```python
from build123d import *

# Parameters (mm, degrees)
SKETCH_1_W           = 42.7
SKETCH_1_H           = 21
SKETCH_1_R           = 1.5
EXTRUDE_1_DEPTH      = 2
SKETCH_2_R           = 1.25
SKETCH_2_R_2         = 3
EXTRUDE_2_DEPTH      = 2
EXTRUDE_3_DEPTH      = 1
EXTRUDE_3_DEPTH_BACK = 3
SKETCH_3_W           = 42.7
SKETCH_3_H           = 21
SKETCH_4_R           = 10.5
SKETCH_4_R_2         = 1.5
EXTRUDE_4_DEPTH      = 1
FILLET_1_R           = 3
FILLET_2_R           = 5
CUT_EXTRUDE_START    = -4
SKETCH_6_R           = 1.5
CUT_EXTRUDE_1_DEPTH  = 4


with BuildPart() as part:
    # 草图1 → 凸台-拉伸1 (new body)
    with BuildSketch(Plane(origin=(0, 0, 0), x_dir=(1, 0, 0), z_dir=(0, 1, 0))):
        Rectangle(SKETCH_1_W, SKETCH_1_H)
        with Locations(Location((7.5, 5, 0), (0, 0, 270))):
            Circle(SKETCH_1_R, mode=Mode.SUBTRACT)
        with Locations(Location((7.5, -5, 0), (0, 0, 90))):
            Circle(SKETCH_1_R, mode=Mode.SUBTRACT)
        with Locations(Location((-7.5, -5, 0), (0, 0, 270))):
            Circle(SKETCH_1_R, mode=Mode.SUBTRACT)
        with Locations(Location((-7.5, 5, 0), (0, 0, 90))):
            Circle(SKETCH_1_R, mode=Mode.SUBTRACT)
        with BuildLine():
            Line((8.017950723, 1.550908082), (12.912587519, 1.550908082))
            ThreePointArc((12.912587519, 1.550908082), (14.126270768, 1.145131224), (14.697546856, 0))
            ThreePointArc((14.697546856, 0), (14.126270768, -1.145131224), (12.912587519, -1.550908082))
            Line((12.912587519, -1.550908082), (8.017950723, -1.550908082))
            add(Edge.make_bspline(
                [(0, -7.407271614), (2.092471107, -7.358009404), (3.043739342, -2.951912586), (6.007732496, -1.626733157), (8.017950723, -1.550908082)],
                knots=[0, 0, 0, 0, 0.496822763, 1, 1, 1, 1], degree=3))
            add(Edge.make_bspline(
                [(0, -7.407271614), (-2.092471107, -7.358009404), (-3.043739342, -2.951912586), (-6.007732496, -1.626733157), (-8.017950723, -1.550908082)],
                knots=[0, 0, 0, 0, 0.496822763, 1, 1, 1, 1], degree=3))
            Line((-8.017950723, -1.550908082), (-12.912587519, -1.550908082))
            ThreePointArc((-12.912587519, -1.550908082), (-14.126270768, -1.145131224), (-14.697546856, 0))
            ThreePointArc((-14.697546856, 0), (-14.126270768, 1.145131224), (-12.912587519, 1.550908082))
            Line((-12.912587519, 1.550908082), (-8.017950723, 1.550908082))
            add(Edge.make_bspline(
                [(0, 7.407271614), (-2.092471107, 7.358009404), (-3.043739342, 2.951912586), (-6.007732496, 1.626733157), (-8.017950723, 1.550908082)],
                knots=[0, 0, 0, 0, 0.496822763, 1, 1, 1, 1], degree=3))
            add(Edge.make_bspline(
                [(0, 7.407271614), (2.092471107, 7.358009404), (3.043739342, 2.951912586), (6.007732496, 1.626733157), (8.017950723, 1.550908082)],
                knots=[0, 0, 0, 0, 0.496822763, 1, 1, 1, 1], degree=3))
        make_face(mode=Mode.SUBTRACT)
    extrude(amount=EXTRUDE_1_DEPTH)

    # 草图2 → 凸台-拉伸2 (add)
    with BuildSketch(Plane.ZY.offset(21.35)):
        with BuildLine():
            Line((-10.5, 2), (-10.5, 32))
            ThreePointArc((-10.5, 32), (0, 42.5), (10.5, 32))
            Line((10.5, 32), (10.5, 2))
            Line((10.5, 2), (-10.5, 2))
        make_face()
        with Locations((0, 24.65)):
            Circle(SKETCH_2_R, mode=Mode.SUBTRACT)
        with Locations((-7.35, 32)):
            Circle(SKETCH_2_R, mode=Mode.SUBTRACT)
        with Locations((0, 39.35)):
            Circle(SKETCH_2_R, mode=Mode.SUBTRACT)
        with Locations((7.35, 32)):
            Circle(SKETCH_2_R, mode=Mode.SUBTRACT)
        with Locations((0, 32)):
            Circle(SKETCH_2_R_2, mode=Mode.SUBTRACT)
    extrude_2 = extrude(amount=-EXTRUDE_2_DEPTH)

    # 镜向1: 凸台-拉伸2 across plane
    add(extrude_2.mirror(Plane(origin=(0, 0, 0), x_dir=(0, 0, 1), z_dir=(1, 0, 0))))

    # 草图3 → 凸台-拉伸3 (add, two sides: drawn at the far end of the back side and taken through both)
    with BuildSketch(Plane.XZ.offset(-EXTRUDE_3_DEPTH_BACK)):
        Rectangle(SKETCH_3_W, SKETCH_3_H)
    extrude(amount=EXTRUDE_3_DEPTH + EXTRUDE_3_DEPTH_BACK)

    # 草图4 → 凸台-拉伸4 (add)
    with BuildSketch(Plane.XZ.offset(1)):
        with Locations(Location((0, 0, 0), (0, 0, 270))):
            Circle(SKETCH_4_R)
        with Locations(Location((0, 7, 0), (0, 0, 270))):
            Circle(SKETCH_4_R_2, mode=Mode.SUBTRACT)
        with Locations(Location((0, -7, 0), (0, 0, 270))):
            Circle(SKETCH_4_R_2, mode=Mode.SUBTRACT)
    extrude(amount=EXTRUDE_4_DEPTH)

    # 圆角1
    fillet_1_edges = [part.edges().sort_by_distance(p)[0] for p in [
        (19.35, 3, 0),
        (-19.35, 3, 0),
    ]]
    fillet(fillet_1_edges, radius=FILLET_1_R)

    # 圆角2
    fillet_2_edges = [part.edges().sort_by_distance(p)[0] for p in [
        (-21.35, -1, 0),
        (21.35, -1, 0),
    ]]
    fillet(fillet_2_edges, radius=FILLET_2_R)

    # 草图6 → 切除-拉伸1 (cut)
    with BuildSketch(Plane.XZ.offset(1).offset(CUT_EXTRUDE_START)):
        with Locations(Location((0, 7, 0), (0, 0, 270))):
            Circle(SKETCH_6_R)
        with Locations(Location((0, -7, 0), (0, 0, 270))):
            Circle(SKETCH_6_R)
    extrude(amount=CUT_EXTRUDE_1_DEPTH, mode=Mode.SUBTRACT)


solid = part.part
```
Geometry check sheet. Reference: the model listing, model coordinates, mm. A direction names the side the tool comes from. Coordinates: 2 decimals unless noted, no trailing zeros. Order: outer loops, then holes, each group sorted by start corner. A loop starts at its lowest first (then second) coordinate and runs counter-clockwise, first axis right, second up.
Item 1: Section check A-A (y = 24.65). Enter the section's corners in (x, z), plus the area to 3 significant figures.
Item 2: Section check B-B (y = 19.5). Enter the section's corners in (x, z).
Item 3: Section check C-C (z = 7). Enter the section's corners in (x, y), plus the area to 3 significant figures.
Item 4: Scan lines: line 1 along X through (y, z) = (27, -7.75); line 2 along Y through (x, z) = (-9, -6.25); line 3 along Y through (x, z) = (-4, 2.75). Record each from-to range of solid material in increasing order.
Item 5: Mould release check, pull along Y, two halves, no side actions. Record for faces 1 (the cylindrical face through (20.36, 38.13, -0.27)), 2 (the flat face through (-12, -1, 0)), 3 (the cylindrical face through (-20.4, 42.5, -0.2)): released by +Y, released by -Y, zero draft, split by the parting line, or undercut.
Item 6: Depth check by flat-ended pin: pin 1 (6 mm diameter, centred on x = 3, z = -1.5, fed in from +Y); pin 2 (10 mm diameter, centred on x = -12.5, z = 8, fed in from +Y). Enter the tip coordinate at first touch or a pass-through.
Item 7: Section check D-D (x = -4.5). Enter the section's corners in (y, z), plus the area to 3 significant figures.
Item 8: Tool access check on faces 4 (the flat face through (12, -1, 0)), 5 (the cylindrical face through (3.2, -1.5, -10)), 6 (the cylindrical face through (18.49, 3.9, -0.15)), 7 (the flat face through (1, 2, -10.5)), 8 (the cylindrical face through (-20.36, 32.05, -8.6)). Record the directions out of +Z, -Z, +X, -X, +Y, -Y that give a thin tool (end or side, any length) a straight path to the whole face; none if there is none.
Check sheet entries:
1. outline: (-21.35, -10.5) - (-19.35, -10.5) - (-19.35, -1.25) - (-21.35, -1.25) - close; (-21.35, 1.25) - (-19.35, 1.25) - (-19.35, 10.5) - (-21.35, 10.5) - close; (19.35, -10.5) - (21.35, -10.5) - (21.35, -1.25) - (19.35, -1.25) - close; (19.35, 1.25) - (21.35, 1.25) - (21.35, 10.5) - (19.35, 10.5) - close
1. area: 74.0 mm2
2. outline: (-21.35, -10.5) - (-19.35, -10.5) - (-19.35, 10.5) - (-21.35, 10.5) - close; (19.35, -10.5) - (21.35, -10.5) - (21.35, 10.5) - (19.35, 10.5) - close
3. outline: (-21.35, 4) arc R5 ccw to (-16.35, -1) - (-7.83, -1) - (-7.83, -2) - (-1.5, -2) - (-1.5, 3) - (-16.35, 3) arc R3 cw to (-19.35, 6) - (-19.35, 30.8) - (-21.35, 30.8) - close; (-21.35, 33.2) - (-19.35, 33.2) - (-19.35, 39.83) - (-21.35, 39.83) - close; (1.5, -2) - (7.83, -2) - (7.83, -1) - (16.35, -1) arc R5 ccw to (21.35, 4) - (21.35, 30.8) - (19.35, 30.8) - (19.35, 6) arc R3 cw to (16.35, 3) - (1.5, 3) - close; (19.35, 33.2) - (21.35, 33.2) - (21.35, 39.83) - (19.35, 39.83) - close
3. area: 302 mm2
4. line 1: x = -21.35 to -19.35, 19.35 to 21.35
4. line 2: y = -1 to 3
4. line 3: y = -2 to 3
5. face 1: undercut
5. face 2: released by -Y
5. face 3: released by +Y
6. pin 1: stops at y = 3
6. pin 2: stops at y = 3.23
7. outline: (-2, -9.49) - (-1, -9.49) - (-1, -10.5) - (3, -10.5) - (3, 10.5) - (-1, 10.5) - (-1, 9.49) - (-2, 9.49) - close
7. area: 103 mm2
8. face 4: +X, -Y
8. face 5: -Y
8. face 6: +Z, -Z, +Y
8. face 7: -Z, +X, -X, +Y, -Y
8. face 8: +X, -X
